from build123d import *

# Parameters (mm, degrees)
BOSS_EXTRUDE1_DEPTH = 60
SKETCH2_R           = 20
SKETCH2_R_2         = 19
CUT_EXTRUDE1_DEPTH  = 10
SKETCH3_R           = 2
CUT_EXTRUDE2_DEPTH  = 10


with BuildPart() as part:
    # Sketch1 → Boss-Extrude1 (new body)
    with BuildSketch(Plane.XY):
        with BuildLine():
            Line((-24.827586207, 75.25862069), (-22.827586207, 75.25862069))
            Line((-22.827586207, 75.25862069), (-22.827586207, -12.74137931))
            ThreePointArc((-22.827586207, -12.74137931), (-19.898654019, -19.812447122), (-12.827586207, -22.74137931))
            Line((-12.827586207, -22.74137931), (55.172413793, -22.74137931))
            Line((55.172413793, -22.74137931), (55.172413793, -24.74137931))
            Line((55.172413793, -24.74137931), (-14.827586207, -24.74137931))
            ThreePointArc((-14.827586207, -24.74137931), (-21.898654019, -21.812447122), (-24.827586207, -14.74137931))
            Line((-24.827586207, -14.74137931), (-24.827586207, 75.25862069))
        make_face()
    extrude(amount=BOSS_EXTRUDE1_DEPTH)

    # Sketch2 → Cut-Extrude1 (cut)
    with BuildSketch(Plane(origin=(-22.827586207, 0, 0), x_dir=(0, 0, -1), z_dir=(1, 0, 0))):
        with Locations((-30, 12.25862069)):
            Circle(SKETCH2_R)
        with Locations((-30, 52.25862069)):
            Circle(SKETCH2_R_2)
    extrude(amount=-CUT_EXTRUDE1_DEPTH, mode=Mode.SUBTRACT)

    # Sketch3 → Cut-Extrude2 (cut)
    with BuildSketch(Plane(origin=(0, -22.74137931, 0), x_dir=(1, 0, 0), z_dir=(0, 1, 0))):
        with Locations((25.172413793, -30)):
            Circle(SKETCH3_R)
    extrude(amount=-CUT_EXTRUDE2_DEPTH, mode=Mode.SUBTRACT)


solid = part.part
Verification items for the finished model (mm, model axes). A direction names the side the tool comes from. Give positions to 0.01 mm unless a question says otherwise; leave off trailing zeros. Write each loop counter-clockwise with the first axis right and the second up, starting at its lowest first coordinate (ties: lowest second). Pieces come first, ordered by that corner, then holes. Notation, with made-up numbers: (49, 41) -> (70, 41) arc R18 ccw to (70, 63) -> close; hole circle Ø1 at (-34.5, -33). An arc over 180 degrees is marked (long way). Use CSV: the item, a comma, the result in double quotes.
(1) Sectioned sample at B-B (y = 51). Record the cut outline in (x, z).
Derived:
outline,"(-24.83, 0) -> (-22.83, 0) -> (-22.83, 11.04) -> (-24.83, 11.04) -> close; (-24.83, 48.96) -> (-22.83, 48.96) -> (-22.83, 60) -> (-24.83, 60) -> close"
(2) Sectioned sample at C-C (z = 44.5). Record the cut outline in (x, y), plus the area to 3 significant figures.
Derived:
outline,"(-24.83, -14.74) arc R10 ccw to (-14.83, -24.74) -> (55.17, -24.74) -> (55.17, -22.74) -> (-12.83, -22.74) arc R10 cw to (-22.83, -12.74) -> (-22.83, -1.52) -> (-24.83, -1.52) -> close; (-24.83, 26.03) -> (-22.83, 26.03) -> (-22.83, 39.98) -> (-24.83, 39.98) -> close; (-24.83, 64.54) -> (-22.83, 64.54) -> (-22.83, 75.26) -> (-24.83, 75.26) -> close"
area,"252 mm^2"
(3) Material ranges on L1, parallel to Y at x = -24, z = 30; L2, parallel to Y at x = 42, z = 17.5; L3, parallel to X at y = -12.5, z = 31.5, recorded low to high.
Derived:
L1,"y = -18.72 to -7.74, 32.26 to 33.26, 71.26 to 75.26"
L2,"y = -24.74 to -22.74"
L3,"x = -24.83 to -22.83"
(4) Sectioned sample at D-D (x = 29.5). Record the cut outline in (y, z), plus the area to 3 significant figures.
Derived:
outline,"(-24.74, 0) -> (-22.74, 0) -> (-22.74, 60) -> (-24.74, 60) -> close"
area,"120 mm^2"
(5) Release check for a two-part mould opening along Y. For faces 1 (the flat face through (21, -24.741, 30)), 2 (the cylindrical face through (26.1, -23.73, 31.77)), 3 (the cylindrical face through (-23.814, 4.599, 11.525)) record: +Y half, -Y half, draft (parallel to the pull), parting line (faces both ways), or undercut.
Derived:
face 1,"-Y half"
face 2,"draft"
face 3,"undercut"
(6) Set-up check for faces 4 (the cylindrical face through (-21.82, -21.89, 29.58)), 5 (the flat face through (21, -22.741, 30)): record each of +Z, -Z, +X, -X, +Y, -Y from which the full face is reachable in a straight line by a thin tool's end or side.
Derived:
face 4,"+Z, -Z, -X, -Y"
face 5,"+Z, -Z, +X, +Y"
(7) Sectioned sample at A-A (z = 30). Record the cut outline in (x, y), plus the area to 3 significant figures.
Derived:
outline,"(-24.83, -14.74) arc R10 ccw to (-14.83, -24.74) -> (23.17, -24.74) -> (23.17, -22.74) -> (-12.83, -22.74) arc R10 cw to (-22.83, -12.74) -> (-22.83, -7.74) -> (-24.83, -7.74) -> close; (-24.83, 32.26) -> (-22.83, 32.26) -> (-22.83, 33.26) -> (-24.83, 33.26) -> close; (-24.83, 71.26) -> (-22.83, 71.26) -> (-22.83, 75.26) -> (-24.83, 75.26) -> close; (27.17, -24.74) -> (55.17, -24.74) -> (55.17, -22.74) -> (27.17, -22.74) -> close"
area,"192 mm^2"
(8) Go/stop test with flat-tipped pins: pin 1 (3 mm diameter, centred on y = -3, z = 21.5, fed in from -X); pin 2 (5 mm diameter, centred on x = 27, z = 18.5, fed in from +Y). Record where each tip stops, or that it passes through.
Derived:
pin 1,"passes through"
pin 2,"stops at y = -22.74"
